from build123d import *

# Parameters (mm, degrees)
BOSS_EXTRUDE2_DEPTH = 50.8
SKETCH4_R           = 3.175
SKETCH4_R_2         = 3.96875
CUT_EXTRUDE1_DEPTH  = 51.165
SKETCH5_R           = 3.175
CUT_EXTRUDE2_DEPTH  = 4.175
SKETCH4_3_R         = 4.7625
SKETCH4_3_R_2       = 3.96875
CUT_EXTRUDE3_DEPTH  = 3.175
SKETCH6_R           = 4.7625
SKETCH6_R_2         = 3.96875
CUT_EXTRUDE4_DEPTH  = 3.175
FILLET1_R           = 12.7
FILLET2_R           = 3.175
FILLET3_R           = 8.89


with BuildPart() as part:
    # Sketch3 → Boss-Extrude2 (new body)
    with BuildSketch(Plane.XY):
        Polygon((-34.6075, 0), (34.6075, 0), (34.6075, 3.175), (15.5575, 3.175), (15.5575, 31.75), (10.795, 31.75), (10.795, 3.175), (-10.795, 3.175), (-10.795, 31.75), (-15.5575, 31.75), (-15.5575, 3.175), (-34.6075, 3.175), align=None)
    extrude(amount=BOSS_EXTRUDE2_DEPTH)

    # Sketch4 → Cut-Extrude1 (cut, through all)
    with BuildSketch(Plane.ZY.offset(15.5575)):
        with Locations((8.89, 15.875)):
            Circle(SKETCH4_R)
        with Locations((41.91, 15.875)):
            Circle(SKETCH4_R)
        with Locations((25.4, 22.225)):
            Circle(SKETCH4_R_2)
    extrude(amount=-CUT_EXTRUDE1_DEPTH, mode=Mode.SUBTRACT)

    # Sketch5 → Cut-Extrude2 (cut, through all)
    with BuildSketch(Plane(origin=(0, 3.175, 0), x_dir=(1, 0, 0), z_dir=(0, 1, 0))):
        with Locations((-25.0825, -38.1)):
            Circle(SKETCH5_R)
        with Locations((-25.0825, -12.7)):
            Circle(SKETCH5_R)
        with Locations((25.0825, -12.7)):
            Circle(SKETCH5_R)
        with Locations((25.0825, -38.1)):
            Circle(SKETCH5_R)
    extrude(amount=-CUT_EXTRUDE2_DEPTH, mode=Mode.SUBTRACT)

    # Sketch4_3 → Cut-Extrude3 (cut)
    with BuildSketch(Plane.ZY.offset(15.5575)):
        with Locations((25.4, 22.225)):
            Circle(SKETCH4_3_R)
        with Locations((25.4, 22.225)):
            Circle(SKETCH4_3_R_2, mode=Mode.SUBTRACT)
    extrude(amount=-CUT_EXTRUDE3_DEPTH, mode=Mode.SUBTRACT)

    # Sketch6 → Cut-Extrude4 (cut)
    with BuildSketch(Plane(origin=(15.5575, 0, 0), x_dir=(0, 0, -1), z_dir=(1, 0, 0))):
        with Locations((-25.4, 22.225)):
            Circle(SKETCH6_R)
        with Locations((-25.4, 22.225)):
            Circle(SKETCH6_R_2, mode=Mode.SUBTRACT)
    extrude(amount=-CUT_EXTRUDE4_DEPTH, mode=Mode.SUBTRACT)

    # Fillet1
    fillet1_edges = [part.edges().sort_by_distance(p)[0] for p in [
        (34.6075, 1.5875, 50.8),
        (34.6075, 1.5875, 0),
        (-34.6075, 1.5875, 0),
        (-34.6075, 1.5875, 50.8),
    ]]
    fillet(fillet1_edges, radius=FILLET1_R)

    # Fillet2
    fillet2_edges = [part.edges().sort_by_distance(p)[0] for p in [
        (-15.5575, 3.175, 25.4),
        (-10.795, 3.175, 25.4),
        (10.795, 3.175, 25.4),
        (15.5575, 3.175, 25.4),
    ]]
    fillet(fillet2_edges, radius=FILLET2_R)

    # Fillet3
    fillet3_edges = [part.edges().sort_by_distance(p)[0] for p in [
        (-13.17625, 31.75, 0),
        (13.17625, 31.75, 0),
        (13.17625, 31.75, 50.8),
        (-13.17625, 31.75, 50.8),
    ]]
    fillet(fillet3_edges, radius=FILLET3_R)


solid = part.part
The listing builds one solid part. Answer for the finished solid, in the listing's coordinates (mm). A direction names the side the tool comes from. Coordinates: 2 decimals unless noted, no trailing zeros. Order: outer loops, then holes, each group sorted by start corner. A loop starts at its lowest first (then second) coordinate and runs counter-clockwise, first axis right, second up. Notation, with made-up numbers: (16.25, 47) -> (43.25, 47) arc R27 ccw to (43.25, 86) -> close; hole circle Ø10 at (-25.75, 22.25). An arc over 180 degrees is marked (long way). Answer in a Markdown table with one row per item. Add a question column.
Item 1: Find section A-A (z = 25.4). State how many separate pieces and enclosed holes the cut face has, then the cut area to 3 significant figures.
Item 2: Which of the six approach directions +Z, -Z, +X, -X, +Y, -Y give full straight-line access (tool end or side, diameter ignored) to faces 4 (the face through (15.558, 16, 25)), 5 (the face through (-10.795, 16, 25)), 6 (the face through (-13.99, 26.24, 27.96))?
Item 3: Determine the mould class of faces 1 (the face through (11.58, 19.81, 22.25)), 2 (the face through (30.986, 1.61, 46.981)), 3 (the face through (16.51, 4.08, 25.76)) for opening direction Y: +Y half, -Y half, draft (parallel to the pull), parting line (faces both ways), or undercut.
Item 4: Find the intervals of material crossed by L1, parallel to X at y = 2.55, z = 12.7; L2, parallel to X at y = 25.5, z = 5 (1 decimal); L3, parallel to Y at x = -14, z = 8.89, in increasing order. Write a range as from..to.
Item 5: Each of these flat-tipped pins is pushed along its axis until it touches: P1, Ø1.5, axis at y = 18, z = 45, coming from the -X side; P2, Ø5, axis at y = 15.875, z = 8.89, coming from the -X side; P3, Ø10, axis at x = -26, y = 7, coming from the -Z side; P4, Ø7.5, axis at y = 16, z = 22.5, coming from the +X side. Where does it stop, or does it pass through?
Item 6: Find section C-C (x = -6.5). Write down the section's boundary in (y, z) (3 decimals), then the cut area to 3 significant figures.
Item 7: Find section B-B (y = 14). Write down the section's boundary in (x, z) (1 decimal), then the cut area to 3 significant figures.
Result set:
| question | item | result |
|---|---|---|
| 1 | separate pieces | 3 |
| 1 | enclosed holes | 0 |
| 1 | area | 415 mm² |
| 2 | face 4 | +Z, -Z, +X, +Y |
| 2 | face 5 | +Z, -Z, +Y |
| 2 | face 6 | -X |
| 3 | face 1 | undercut |
| 3 | face 2 | draft |
| 3 | face 3 | +Y half |
| 4 | L1 | x = -34.61..-28.26, -21.91..21.91, 28.26..34.61 |
| 4 | L2 | x = -15.6..-10.8, 10.8..15.6 |
| 4 | L3 | y = 0..12.7, 19.05..31.75 |
| 5 | P1 | stops at x = -15.56 |
| 5 | P2 | passes through |
| 5 | P3 | stops at z = 0.03 |
| 5 | P4 | stops at x = 15.56 |
| 6 | outline | (0, 0) -> (3.175, 0) -> (3.175, 50.8) -> (0, 50.8) -> close |
| 6 | area | 161 mm² |
| 7 | outline | (-15.6, 0) -> (-10.8, 0) -> (-10.8, 6.3) -> (-15.6, 6.3) -> close; (-15.6, 11.5) -> (-10.8, 11.5) -> (-10.8, 39.3) -> (-15.6, 39.3) -> close; (-15.6, 44.5) -> (-10.8, 44.5) -> (-10.8, 50.8) -> (-15.6, 50.8) -> close; (10.8, 0) -> (15.6, 0) -> (15.6, 6.3) -> (10.8, 6.3) -> close; (10.8, 11.5) -> (15.6, 11.5) -> (15.6, 39.3) -> (10.8, 39.3) -> close; (10.8, 44.5) -> (15.6, 44.5) -> (15.6, 50.8) -> (10.8, 50.8) -> close |
| 7 | area | 386 mm² |
